Work out the finished part from the listing and answer in its coordinate system (mm). Face numbers are marked on the shaded views. A direction names the side the tool comes from. Coordinates: 2 decimals unless noted, no trailing zeros. Order: outer loops, then holes, each group sorted by start corner. A loop starts at its lowest first (then second) coordinate and runs counter-clockwise, first axis right, second up. Notation, with made-up numbers: M -38.75,5.25 L 14.25,5.25 A16 cw 14.25,18.25 Z; hole C -20,-7 d1. An arc over 180 degrees is marked long. Use a Markdown table: item, result.
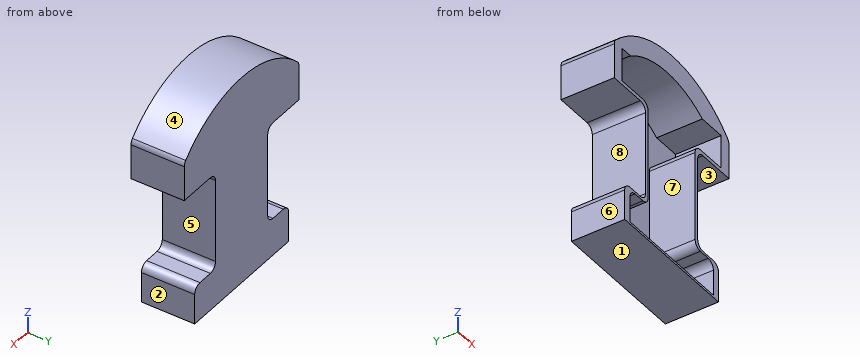
from build123d import *

# Parameters (mm, degrees)
BOSS_EXTRUDE1_DEPTH = 70
FILLET3_R           = 10
BOSS_EXTRUDE2_DEPTH = 10
FILLET4_R           = 10


with BuildPart() as part:
    # Sketch1 → Boss-Extrude1 (new body)
    with BuildSketch(Plane(origin=(0, 0, 0), x_dir=(1, 0, 0), z_dir=(0, 1, 0))):
        with BuildLine():
            Line((-90, 17.965988739), (90, 17.965988739))
            Line((90, 17.965988739), (90, -32.034011261))
            Line((90, -32.034011261), (50, -32.034011261))
            Line((50, -32.034011261), (50, -162.034011261))
            Line((50, -162.034011261), (110, -162.034011261))
            Line((110, -162.034011261), (110, -212.034011261))
            ThreePointArc((110, -212.034011261), (0, -260.808853853), (-110, -212.034011261))
            Line((-110, -212.034011261), (-110, -162.034011261))
            Line((-110, -162.034011261), (-50, -162.034011261))
            Line((-50, -162.034011261), (-50, -32.034011261))
            Line((-50, -32.034011261), (-90, -32.034011261))
            Line((-90, -32.034011261), (-90, 17.965988739))
        make_face()
        with BuildLine():
            Line((-80, 14.965988739), (80, 14.965988739))
            Line((80, 14.965988739), (80, -29.034011261))
            Line((80, -29.034011261), (45, -29.034011261))
            Line((45, -29.034011261), (45, -167.034011261))
            Line((45, -167.034011261), (95, -167.034011261))
            Line((95, -167.034011261), (95, -211.241666668))
            Line((95, -211.241666668), (58.77564579, -211.241666668))
            ThreePointArc((58.77564579, -211.241666668), (-10.047427033, -232.545270894), (-78.870499857, -211.241666668))
            Line((-78.870499857, -211.241666668), (-95, -211.241666668))
            Line((-95, -211.241666668), (-95, -167.034011261))
            Line((-95, -167.034011261), (-45, -167.034011261))
            Line((-45, -167.034011261), (-45, -29.034011261))
            Line((-45, -29.034011261), (-80, -29.034011261))
            Line((-80, -29.034011261), (-80, 14.965988739))
        make_face(mode=Mode.SUBTRACT)
    extrude(amount=BOSS_EXTRUDE1_DEPTH)

    # Fillet3
    fillet3_edges = [part.edges().sort_by_distance(p)[0] for p in [
        (-90, 35, 32.034011261),
    ]]
    fillet(fillet3_edges, radius=FILLET3_R)

    # Sketch9 → Boss-Extrude2 (add)
    with BuildSketch(Plane(origin=(0, 70, 0), x_dir=(1, 0, 0), z_dir=(0, 1, 0))):
        with BuildLine():
            Line((-90, 17.965988739), (-90, -22.034011261))
            ThreePointArc((-90, -22.034011261), (-87.071067812, -29.105079073), (-80, -32.034011261))
            Line((-80, -32.034011261), (-50, -32.034011261))
            Line((-50, -32.034011261), (-50, -162.034011261))
            Line((-50, -162.034011261), (-110, -162.034011261))
            Line((-110, -162.034011261), (-110, -212.034011261))
            ThreePointArc((-110, -212.034011261), (0, -260.808853853), (110, -212.034011261))
            Line((110, -212.034011261), (110, -162.034011261))
            Line((110, -162.034011261), (50, -162.034011261))
            Line((50, -162.034011261), (50, -32.034011261))
            Line((50, -32.034011261), (90, -32.034011261))
            Line((90, -32.034011261), (90, 17.965988739))
            Line((90, 17.965988739), (-90, 17.965988739))
        make_face()
    extrude(amount=-BOSS_EXTRUDE2_DEPTH)

    # Fillet4
    fillet4_edges = [part.edges().sort_by_distance(p)[0] for p in [
        (-45, 30, 167.034011261),
        (-45, 30, 29.034011261),
        (-80, 30, 29.034011261),
        (90, 35, 32.034011261),
        (50, 35, 32.034011261),
        (50, 35, 162.034011261),
        (110, 35, 212.034011261),
        (-110, 35, 212.034011261),
        (-50, 35, 162.034011261),
        (-50, 35, 32.034011261),
        (80, 30, 29.034011261),
        (45, 30, 29.034011261),
        (45, 30, 167.034011261),
    ]]
    fillet(fillet4_edges, radius=FILLET4_R)


solid = part.part
(1) A cutting plane is placed at C-C (z = 242). Determine the outline of the cut face in (x, y), then the cut area to 3 significant figures.
Conclusion:
| item | result |
|---|---|
| outline | M -72.32,0 L 72.32,0 L 72.32,70 L -72.32,70 Z |
| area | 10,100 mm2 |
(2) A cutting plane is placed at A-A (z = 170.5). Determine the outline of the cut face in (x, y), then the cut area to 3 significant figures.
Conclusion:
| item | result |
|---|---|
| outline | M -110,0 L -95,0 L -95,60 L 95,60 L 95,0 L 110,0 L 110,70 L -110,70 Z |
| area | 4,000 mm2 |
(3) Given P1, Ø12, axis at x = 36, z = 36.5, coming from the -Y side; P2, Ø2, axis at x = 76, y = 10, coming from the +Z side; P3, Ø5, axis at x = 14.5, y = 55.5, coming from the +Z side; P4, Ø5, axis at x = -91, y = 27, coming from the -Z side, each flat-ended and moving along its own axis, determine where each tip first touches the part or whether it passes through.
Conclusion:
| item | result |
|---|---|
| P1 | y = 60 |
| P2 | z = 240.47 |
| P3 | z = 260.32 |
| P4 | z = -17.97 |
(4) Determine the mould class of the marked faces 1, 2, 3 and 4 for opening direction Z: pulls with the +Z half, pulls with the -Z half, needs draft (parallel to the pull), parting line crosses it, or undercut.
Conclusion:
| item | result |
|---|---|
| face 1 | pulls with the -Z half |
| face 2 | needs draft |
| face 3 | undercut |
| face 4 | pulls with the +Z half |
(5) Straight lines are drawn through the part: L1, parallel to X at y = 44, z = 83; L2, parallel to Z at x = 47, y = 9.5; L3, parallel to Z at x = 73, y = 57. For each, find the intervals that lie inside material, in ascending order.
Conclusion:
| item | result |
|---|---|
| L1 | -50 to -45, 45 to 50 |
| L2 | -17.97 to -14.97, 33.03 to 163.03, 218.36 to 253.17 |
| L3 | -17.97 to -14.97, 28.57 to 32.03, 162.03 to 167.03, 211.24 to 241.62 |
(6) Which of the six approach directions +Z, -Z, +X, -X, +Y, -Y give full straight-line access (tool end or side, diameter ignored) to the marked faces 5, 6, 7 and 8?
Conclusion:
| item | result |
|---|---|
| face 5 | +X, +Y, -Y |
| face 6 | -Z, -X, +Y, -Y |
| face 7 | -Y |
| face 8 | -X, +Y, -Y |
(7) A cutting plane is placed at B-B (x = -34). Determine the outline of the cut face in (y, z), then the cut area to 3 significant figures.
Conclusion:
| item | result |
|---|---|
| outline | M 0,-17.97 L 70,-17.97 L 70,256.86 L 0,256.86 L 0,230.17 L 60,230.17 L 60,-14.97 L 0,-14.97 Z |
| area | 4,530 mm2 |
